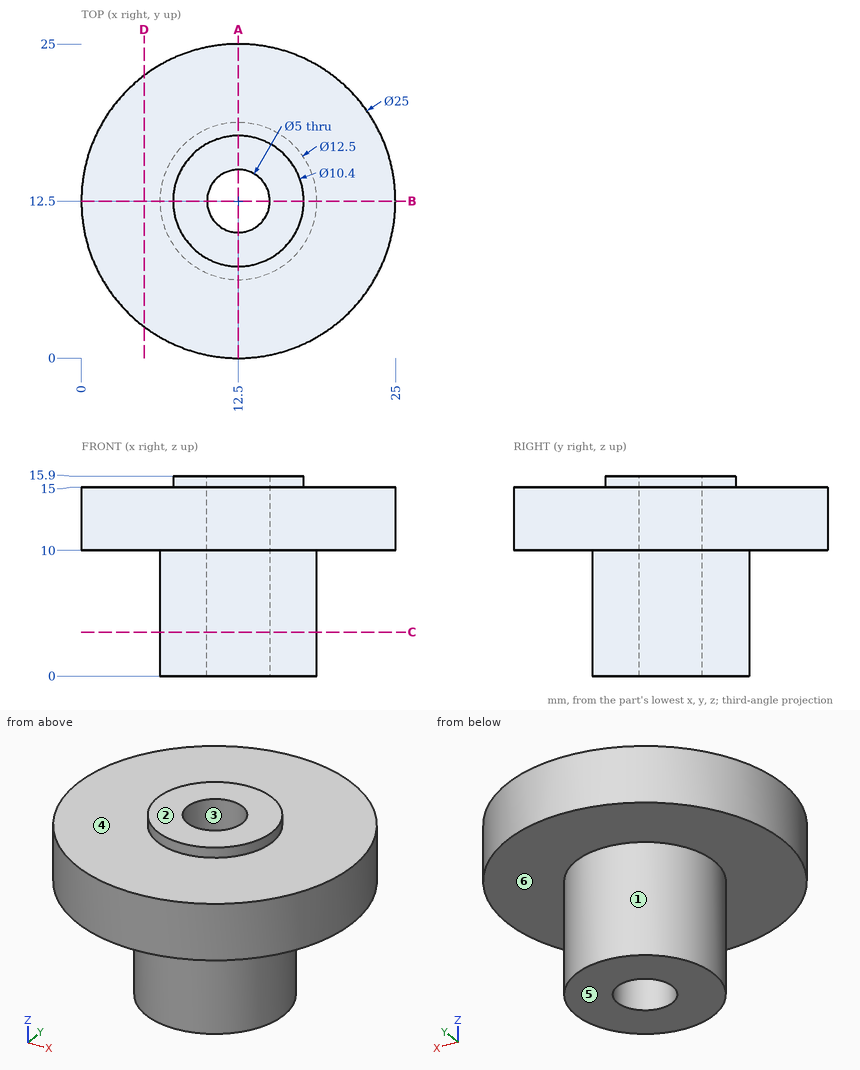
Design review of the part shown in the three views and the two pictorial views. Dimensions are in mm from the part's minimum x, y and z. A direction names the side the tool comes from. Give positions to 0.01 mm unless a question says otherwise; leave off trailing zeros. Write each loop counter-clockwise with the first axis right and the second up, starting at its lowest first coordinate (ties: lowest second). Pieces come first, ordered by that corner, then holes. Notation, with made-up numbers: M 77.25,62 L 136.25,62 A17 cw 136.25,84 Z; hole C -21,69 d5. An arc over 180 degrees is marked long. One line per question, with ' | ' between items. Start each with the question number.
Item 1: Wall thickness on line 1 (Y direction, x = 12.5, z = 7.5); line 2 (Y direction, x = 12.5, z = 12.75); line 3 (Z direction, x = 12.75, y = 5.5): over which ranges is each line inside the solid? List them lowest first. Write a range as from..to.
Item 2: For pin 1 (6 mm diameter, centred on x = 3.5, z = 7.5, fed in from +Y); pin 2 (2 mm diameter, centred on x = 11, y = 22, fed in from +Z); pin 3 (2 mm diameter, centred on y = 6.5, z = 3, fed in from +X), all flat-tipped, find the tip position at first contact; note any pin that passes through.
Item 3: Draft analysis for pull direction Y (two halves, no side actions). For the marked faces 1, 2 and 3, state which applies: released by +Y, released by -Y, zero draft, split by the parting line, or undercut.
Item 4: We need section A-A on x = 12.5. Write out the cut boundary in (y, z), plus the area to 3 significant figures.
Item 5: For the marked faces 4, 5 and 6, list the 3-axis set-ups (+Z, -Z, +X, -X, +Y, -Y) from which the entire face can be reached by the end or side of a thin tool; tool diameter is ignored.
Item 6: We need section D-D on x = 5. Write out the cut boundary in (y, z).
Item 7: We need section C-C on z = 3.5. Write out the cut boundary in (x, y), plus the area to 3 significant figures.
Results found:
1) line 1: y = 6.25..10, 15..18.75 | line 2: y = 0..10, 15..25 | line 3: z = 10..15
2) pin 1: stops at y = 22.62 | pin 2: stops at z = 15 | pin 3: stops at x = 16.25
3) face 1: split by the parting line | face 2: zero draft | face 3: undercut
4) outline: M 0,10 L 6.25,10 L 6.25,0 L 10,0 L 10,15.9 L 7.3,15.9 L 7.3,15 L 0,15 Z; M 15,0 L 18.75,0 L 18.75,10 L 25,10 L 25,15 L 17.7,15 L 17.7,15.9 L 15,15.9 Z | area: 180 mm2
5) face 4: +Z | face 5: -Z, +X, -X, +Y, -Y | face 6: -Z
6) outline: M 2.5,10 L 22.5,10 L 22.5,15 L 2.5,15 Z
7) outline: C 12.5,12.5 d12.5; hole C 12.5,12.5 d5 | area: 103 mm2
